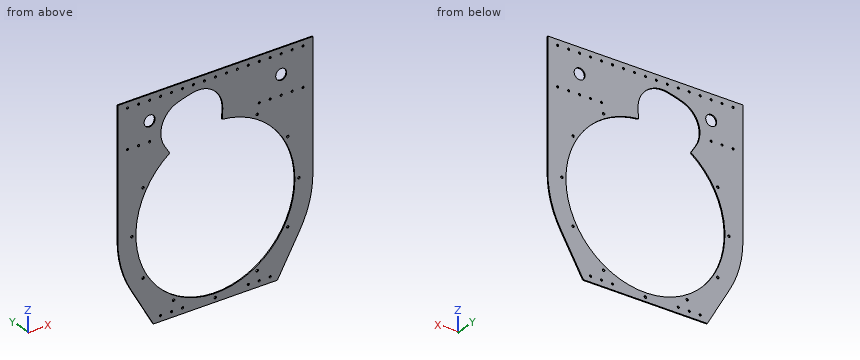
```python
from build123d import *

# Parameters (mm, degrees)
SKETCH1_W               = 539.75
SKETCH1_H               = 495.3
BOSS_EXTRUDE1_DEPTH     = 2.54
SKETCH2_R               = 184.15
CUT_EXTRUDE1_DEPTH      = 467.904666099
CUT_EXTRUDE3_DEPTH      = 443.942729481
CUT_EXTRUDE3_DEPTH_BACK = 443.942729481
SKETCH4_OUTSIDE_W       = 587.882
SKETCH4_OUTSIDE_H       = 631.382
DELETEFACE1_DEPTH       = 2.54
F_8_CLEARANCE_HOLE1_D   = 4.9149
F_10_CLEARANCE_HOLE1_D  = 5.6134
SKETCH10_R              = 12.7
CUT_EXTRUDE4_DEPTH      = 443.942729481


# Read off the part's stored shape, not the designer's step: DeleteFace1
with BuildPart() as part:
    # Sketch1 → Boss-Extrude1 (new body)
    with BuildSketch(Plane(origin=(0, 0, 0), x_dir=(1, 0, 0), z_dir=(0, 1, 0))):
        with Locations((0, 133.35)):
            Rectangle(SKETCH1_W, SKETCH1_H)
    extrude(amount=BOSS_EXTRUDE1_DEPTH)

    # Sketch2 → Cut-Extrude1 (cut, through all)
    with BuildSketch(Plane(origin=(0, 2.54, 0), x_dir=(1, 0, 0), z_dir=(0, 1, 0))):
        with Locations(Location((0, 177.8, 0), (0, 0, 270))):
            Circle(SKETCH2_R)
        with BuildLine():
            Line((195.635138715, 290.75), (99.054025744, 458.033394716))
            Line((99.054025744, 458.033394716), (644.549965459, 478.864376008))
            Line((644.549965459, 478.864376008), (667.56593599, -123.849355899))
            Line((667.56593599, -123.849355899), (225.9, -158.139047855))
            Line((225.9, -158.139047855), (225.9, 177.8))
            ThreePointArc((225.9, 177.8), (218.202644159, 236.267222289), (195.635138715, 290.75))
        make_face()
        with BuildLine():
            Line((-99.054025744, 458.033394716), (-195.635138715, 290.75))
            ThreePointArc((-195.635138715, 290.75), (-218.202644159, 236.267222289), (-225.9, 177.8))
            Line((-225.9, 177.8), (-225.9, -158.139047855))
            Line((-225.9, -158.139047855), (-512.847328359, -198.052843622))
            Line((-512.847328359, -198.052843622), (-480.715151615, 488.522350563))
            Line((-480.715151615, 488.522350563), (-99.054025744, 458.033394716))
        make_face()
    extrude(amount=-CUT_EXTRUDE1_DEPTH, mode=Mode.SUBTRACT)

    # Sketch4 outside → Cut-Extrude3 (cut, two sides: drawn at the far end of the back side and taken through both)
    # profile 1 of 2: a face of its own
    with BuildSketch(Plane(origin=(0, 2.54, 0), x_dir=(1, 0, 0), z_dir=(0, 1, 0)).offset(-CUT_EXTRUDE3_DEPTH_BACK)):
        with Locations((0, 133.35)):
            Rectangle(SKETCH4_OUTSIDE_W, SKETCH4_OUTSIDE_H)
        with BuildLine():
            Line((195.635138715, 290.75), (143.529276921, 381))
            Line((143.529276921, 381), (-143.529276921, 381))
            Line((-143.529276921, 381), (-195.635138715, 290.75))
            ThreePointArc((-195.635138715, 290.75), (-218.202644159, 236.267222289), (-225.9, 177.8))
            Line((-225.9, 177.8), (-225.9, -114.3))
            Line((-225.9, -114.3), (225.9, -114.3))
            Line((225.9, -114.3), (225.9, 177.8))
            ThreePointArc((225.9, 177.8), (218.202644159, 236.267222289), (195.635138715, 290.75))
        make_face(mode=Mode.SUBTRACT)
    # profile 2 of 2: a face of its own
    with BuildSketch(Plane(origin=(0, 2.54, 0), x_dir=(1, 0, 0), z_dir=(0, 1, 0)).offset(-CUT_EXTRUDE3_DEPTH_BACK)):
        with BuildLine():
            Line((17.092062212, -27.00447678), (16.405511664, -13.904311929))
            ThreePointArc((16.405511664, -13.904311929), (12.375480651, -5.272574167), (3.477179505, -1.871356225))
            ThreePointArc((3.477179505, -1.871356225), (-46.5110765, 4.218299387), (-92.847003898, 23.93863093))
            ThreePointArc((-92.847003898, 23.93863093), (-102.253767711, 25.442240361), (-110.059745828, 19.981951687))
            Line((-110.059745828, 19.981951687), (-117.204398469, 8.980151406))
            ThreePointArc((-117.204398469, 8.980151406), (-123.287148558, -40.070635127), (-88.464039092, -75.146703255))
            ThreePointArc((-88.464039092, -75.146703255), (-69.355739516, -81.039143671), (-49.861246452, -85.490290368))
            ThreePointArc((-49.861246452, -85.490290368), (-2.165514952, -72.525079038), (17.092062212, -27.00447678))
        make_face()
    extrude(amount=CUT_EXTRUDE3_DEPTH + CUT_EXTRUDE3_DEPTH_BACK, mode=Mode.SUBTRACT)

    # DeleteFace1 outline → DeleteFace1 (cut)
    with BuildSketch(Plane(origin=(0, 0, 0), x_dir=(1, 0, 0), z_dir=(0, 1, 0))):
        with BuildLine():
            ThreePointArc((-103.099865089, 25.216775763), (-104.333958967, 26.057957355), (-105.561190084, 26.909120064))
            Line((-105.561190084, 26.909120064), (-110.059745828, 19.981951687))
            ThreePointArc((-110.059745828, 19.981951687), (-107.042541375, 23.214587225), (-103.099865089, 25.216775763))
        make_face()
        with BuildLine():
            Line((16.405511664, -13.904311929), (15.973232299, -5.655930266))
            ThreePointArc((15.973232299, -5.655930266), (14.484837621, -5.779443236), (12.995490176, -5.890880925))
            ThreePointArc((12.995490176, -5.890880925), (15.408853729, -9.596165205), (16.405511664, -13.904311929))
        make_face()
    extrude(amount=DELETEFACE1_DEPTH, mode=Mode.SUBTRACT)

    # #8 Clearance Hole1 (through all)
    with Locations(Plane(origin=(0, 2.54, 0), x_dir=(1, 0, 0), z_dir=(0, 1, 0))):
        with Locations((127, -101.6), (101.6, -101.6), (76.2, -101.6), (50.8, -101.6), (25.4, -101.6), (0, -101.6), (-25.4, -101.6), (-50.8, -101.6), (-76.2, -101.6), (-101.6, -101.6), (-127, -101.6), (-152.4, -101.6), (-177.8, -101.6), (-203.2, -101.6), (-152.4, -12.7), (-177.8, -12.7), (-203.2, -12.7), (101.6, -12.7), (127, -12.7), (152.4, -12.7), (152.4, -101.6), (177.8, -101.6), (203.2, -101.6), (203.2, -12.7), (177.8, -12.7), (127, 368.3), (101.6, 368.3), (76.2, 368.3), (-76.2, 368.3), (-101.6, 368.3), (-127, 368.3)):
            Hole(F_8_CLEARANCE_HOLE1_D / 2)

    # #10 Clearance Hole1 (through all)
    with Locations(Plane(origin=(0, 2.54, 0), x_dir=(1, 0, 0), z_dir=(0, 1, 0))):
        with Locations((-167.575915632, 274.55), (-96.75, 345.375915632), (0, 371.3), (96.75, 345.375915632), (167.575915632, 274.55), (193.5, 177.8), (167.575915632, 81.05), (96.75, 10.224084368), (-167.575915632, 81.05), (-193.5, 177.8)):
            Hole(F_10_CLEARANCE_HOLE1_D / 2)

    # Sketch10 → Cut-Extrude4 (cut, through all)
    with BuildSketch(Plane(origin=(0, 2.54, 0), x_dir=(1, 0, 0), z_dir=(0, 1, 0))):
        with Locations(Location((-152.4, -57.15, 0), (0, 0, 270))):
            Circle(SKETCH10_R)
        with Locations(Location((152.4, -57.15, 0), (0, 0, 270))):
            Circle(SKETCH10_R)
    extrude(amount=-CUT_EXTRUDE4_DEPTH, mode=Mode.SUBTRACT)


solid = part.part
```
Can you work these out from the model? Positions are in its coordinate system, mm. Round coordinates to 2 decimals unless told otherwise and drop trailing zeros. Loops run counter-clockwise (first coordinate to the right, second up) from the corner with the lowest first, then second, coordinate; pieces in that order, holes last. Notation, with made-up numbers: (36, 29) -> (88, 29) arc R26 ccw to (88, 46) -> close; hole circle Ø10 at (44.25, 30). An arc over 180 degrees is marked (long way). One line per item, written item: value. Start each with the question number.
1. If I drill on probe 1 along Z at (x, y) = (-203.2, 2); probe 2 along X at (y, z) = (1, -276.5); probe 3 along X at (y, z) = (1, 50.5), over which ranges is the centre line in solid material (lowest first)?
2. For pin 1 (6.5 mm diameter, centred on x = -127, z = 101.6, fed in from -Y), with a flat end and sliding along its axis, tell me the tip position at first contact or that it passes through.
3. If we section it at C-C, the plane y = 1.15: Give the number of separate pieces and of enclosed holes in the cut face, then the cut area to 3 significant figures.
4. If we section it at B-B, the plane z = -69.5: Write out the boundary of the cut face in (x, y).
5. If we section it at A-A, the plane z = -204.5: Write out the boundary of the cut face in (x, y), then the cut area to 3 significant figures.
Calculated:
1. probe 1: z = -276.49 to 10.24, 15.16 to 99.14, 104.06 to 114.3
1. probe 2: x = -203.2 to -169.59, -165.56 to -155.47, 155.47 to 165.56, 169.59 to 203.2
1. probe 3: x = -225.9 to -163.22, -141.58 to -118.49, 13.31 to 141.58, 163.22 to 225.9
2. pin 1: stops at y = 0
3. separate pieces: 1
3. enclosed holes: 44
3. area: 91,900 mm²
4. outline: (-225.9, 0) -> (-148.94, 0) -> (-148.94, 2.54) -> (-225.9, 2.54) -> close; (148.94, 0) -> (225.9, 0) -> (225.9, 2.54) -> (148.94, 2.54) -> close
5. outline: (-224.32, 0) -> (-182.2, 0) -> (-182.2, 2.54) -> (-224.32, 2.54) -> close; (182.2, 0) -> (224.32, 0) -> (224.32, 2.54) -> (182.2, 2.54) -> close
5. area: 214 mm²
